from build123d import *

# Parameters (mm, degrees)
EXTRUDE_1_DEPTH      = 15.2
EXTRUDE_1_DEPTH_BACK = 15.2
SKETCH_1_R           = 1
SKETCH_2_W           = 26.4
SKETCH_2_H           = 30.2
CUT_EXTRUDE_1_DEPTH  = 30.3
CUT_EXTRUDE_2_REACH  = 48.384
EXTRUDE_2_DEPTH      = 2
EXTRUDE_2_DEPTH_BACK = 1.5
SKETCH_4_W           = 45
SKETCH_4_H           = 45
SKETCH_5_R           = 1.5
CUT_EXTRUDE_3_DEPTH  = 3.5


with BuildPart() as part:
    # 草图1 → 凸台-拉伸1 (new, two sides: drawn at the far end of the back side and taken through both)
    with BuildSketch(Plane(origin=(0, 0, 0), x_dir=(0, 0, -1), z_dir=(1, 0, 0)).offset(-EXTRUDE_1_DEPTH_BACK)):
        with BuildLine():
            Line((-6.7, 0), (6.7, 0))
            ThreePointArc((6.7, 0), (7.402943725, 1.697056275), (9.1, 2.4))
            Line((9.1, 2.4), (9.1, 27.4))
            Line((9.1, 27.4), (17.1, 27.4))
            Line((17.1, 27.4), (17.1, 0))
            Line((17.1, 0), (17.1, -4.9))
            Line((17.1, -4.9), (9.1, -4.9))
            Line((9.1, -4.9), (-9.1, -4.9))
            Line((-9.1, -4.9), (-17.1, -4.9))
            Line((-17.1, -4.9), (-17.1, 0))
            Line((-17.1, 0), (-17.1, 27.4))
            Line((-17.1, 27.4), (-9.1, 27.4))
            Line((-9.1, 27.4), (-9.1, 2.4))
            ThreePointArc((-9.1, 2.4), (-7.402943725, 1.697056275), (-6.7, 0))
        make_face()
        with Locations((9.1, 0)):
            Circle(SKETCH_1_R, mode=Mode.SUBTRACT)
        with Locations((-9.1, 0)):
            Circle(SKETCH_1_R, mode=Mode.SUBTRACT)
    extrude(amount=EXTRUDE_1_DEPTH + EXTRUDE_1_DEPTH_BACK)

    # 草图2 → 切除-拉伸1 (cut)
    with BuildSketch(Plane(origin=(0, 27.4, 0), x_dir=(1, 0, 0), z_dir=(0, 1, 0))):
        Rectangle(SKETCH_2_W, SKETCH_2_H)
    extrude(amount=-CUT_EXTRUDE_1_DEPTH, mode=Mode.SUBTRACT)

    # 切除-拉伸2: up to this face of the body (flat: up to its plane)
    cut_extrude_2_end = Plane(part.part.faces().sort_by_distance((0, 11.25, 17.1))[0])
    # 草图3 → 切除-拉伸2 (cut, up to the picked face)
    with BuildSketch(Plane(origin=(0, 0, -17.1), x_dir=(-1, 0, 0), z_dir=(0, 0, -1)), mode=Mode.PRIVATE) as cut_extrude_2_sk1:
        with BuildLine():
            Line((5.280872039, 17.60905008), (5.280872039, 8.98362575))
            ThreePointArc((5.280872039, 8.98362575), (0, 3.702753711), (-5.280872039, 8.98362575))
            Line((-5.280872039, 8.98362575), (-5.280872039, 17.60905008))
            ThreePointArc((-5.280872039, 17.60905008), (0, 22.889922119), (5.280872039, 17.60905008))
        make_face()
    cut_extrude_2_tool1 = split(extrude(cut_extrude_2_sk1.sketch, amount=-CUT_EXTRUDE_2_REACH, mode=Mode.PRIVATE), bisect_by=cut_extrude_2_end, keep=Keep.BOTH, mode=Mode.PRIVATE)
    add(cut_extrude_2_tool1.solids().sort_by(Axis((0, 13.296338, -17.1), (0, 0, 1)))[0], mode=Mode.SUBTRACT)

    # 草图4 → 凸台-拉伸2 (add, two sides: drawn at the far end of the back side and taken through both)
    with BuildSketch(Plane.XZ.offset(4.9).offset(-EXTRUDE_2_DEPTH_BACK)):
        Rectangle(SKETCH_4_W, SKETCH_4_H)
    extrude(amount=EXTRUDE_2_DEPTH + EXTRUDE_2_DEPTH_BACK)

    # 草图5 → 切除-拉伸3 (cut)
    with BuildSketch(Plane(origin=(0, -3.4, 0), x_dir=(1, 0, 0), z_dir=(0, 1, 0))):
        with Locations(Location((-18.679189152, 18.679189152, 0), (0, 0, 270))):
            Circle(SKETCH_5_R)
        with Locations(Location((18.679189152, 18.679189152, 0), (0, 0, 90))):
            Circle(SKETCH_5_R)
        with Locations(Location((-18.679189152, -18.679189152, 0), (0, 0, 90))):
            Circle(SKETCH_5_R)
        with Locations(Location((18.679189152, -18.679189152, 0), (0, 0, 270))):
            Circle(SKETCH_5_R)
    extrude(amount=-CUT_EXTRUDE_3_DEPTH, mode=Mode.SUBTRACT)


solid = part.part
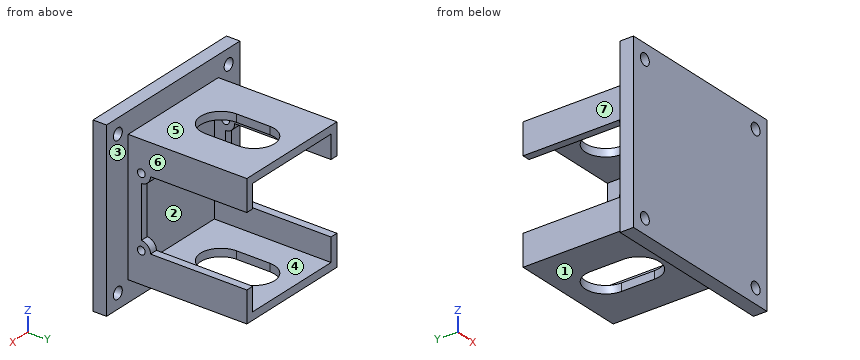
Input: part model. Units: mm. Frame: model coordinates. Face numbers are marked on the shaded views. A direction names the side the tool comes from. Give positions to 0.01 mm unless a question says otherwise; leave off trailing zeros. Order: outer loops, then holes, each group sorted by start corner. A loop starts at its lowest first (then second) coordinate and runs counter-clockwise, first axis right, second up. Notation, with made-up numbers: M 36,-25 L 47,-25 A21 ccw 47,10 Z; hole C 78.5,69.5 d10. An arc over 180 degrees is marked long. Answer as a JSON object with one key per item and string values.
1. Cut plane D-D, the plane x = -6.5. Output: boundary loops of the cut face in (y, z), and give its area (3 significant figures).
Result sheet:
{"outline": "M -6.9,-22.5 L -3.4,-22.5 L -3.4,-17.1 L 27.4,-17.1 L 27.4,-15.1 L -2.9,-15.1 L -2.9,15.1 L 27.4,15.1 L 27.4,17.1 L -3.4,17.1 L -3.4,22.5 L -6.9,22.5 Z", "area": "296 mm²"}
2. First-contact query: P1, Ø8, axis at x = 12, y = 19.5, coming from the +Z side; P2, Ø3, axis at x = 13, z = 3.5, coming from the +Y side; P3, Ø3, axis at y = 0, z = 9.1, coming from the +X side. Flat tips, straight axial feed; report the tip coordinate or a pass-through.
Result sheet:
{"P1": "z = 17.1", "P2": "y = 0", "P3": "x = 15.2"}
3. Pull-direction query (Z, two-part tool) for the marked faces 1, 2 and 3; classes: +Z half, -Z half, draft (parallel to the pull), parting line (faces both ways), or undercut.
Result sheet:
{"face 1": "-Z half", "face 2": "undercut", "face 3": "draft"}
4. Cut plane A-A, the plane x = 0. Output: boundary loops of the cut face in (y, z), and give its area (3 significant figures).
Result sheet:
{"outline": "M -6.9,-22.5 L -3.4,-22.5 L -3.4,-17.1 L 3.7,-17.1 L 3.7,-15.1 L -2.9,-15.1 L -2.9,15.1 L 3.7,15.1 L 3.7,17.1 L -3.4,17.1 L -3.4,22.5 L -6.9,22.5 Z; M 22.89,-17.1 L 27.4,-17.1 L 27.4,-15.1 L 22.89,-15.1 Z; M 22.89,15.1 L 27.4,15.1 L 27.4,17.1 L 22.89,17.1 Z", "area": "219 mm²"}
5. Reachability of the marked faces 4, 5, 6 and 7 from +Z, -Z, +X, -X, +Y, -Y: full face, straight path, thin tool, end or side. Return the list, or none.
Result sheet:
{"face 4": "+Y", "face 5": "+Z, +X, -X, +Y", "face 6": "+Z, -Z, +X, +Y", "face 7": "+Z, -Z, -X, +Y"}
6. Ray query, line 1 (Y direction, x = -14, z = -9); line 2 (Z direction, x = -5.5, y = 11.5); line 3 (X direction, y = 17.5, z = 16). Return the intervals inside material, ascending. Write a range as [from, to].
Result sheet:
{"line 1": "[-6.9, -0.99], [0.99, 2.4]", "line 2": "[-17.1, -15.1], [15.1, 17.1]", "line 3": "[-15.2, -5.28], [5.28, 15.2]"}
7. Cut plane C-C, the plane y = 16. Output: boundary loops of the cut face in (x, z).
Result sheet:
{"outline": "M -15.2,-17.1 L -5.28,-17.1 L -5.28,-15.1 L -13.2,-15.1 L -13.2,-9.1 L -15.2,-9.1 Z; M -15.2,9.1 L -13.2,9.1 L -13.2,15.1 L -5.28,15.1 L -5.28,17.1 L -15.2,17.1 Z; M 5.28,-17.1 L 15.2,-17.1 L 15.2,-9.1 L 13.2,-9.1 L 13.2,-15.1 L 5.28,-15.1 Z; M 5.28,15.1 L 13.2,15.1 L 13.2,9.1 L 15.2,9.1 L 15.2,17.1 L 5.28,17.1 Z"}
8. Cut plane B-B, the plane y = -2. Output: boundary loops of the cut face in (x, z).
Result sheet:
{"outline": "M -15.2,-17.1 L 15.2,-17.1 L 15.2,17.1 L -15.2,17.1 Z; hole M -13.2,-15.1 L 13.2,-15.1 L 13.2,15.1 L -13.2,15.1 Z"}
